Check sheet for the drawn part. Datum: minimum x, y, z corner. Units: mm. Round coordinates to 2 decimals unless told otherwise and drop trailing zeros. Write each loop counter-clockwise with the first axis right and the second up, starting at its lowest first coordinate (ties: lowest second). Pieces come first, ordered by that corner, then holes. Notation, with made-up numbers: M 47,-28.5 L 60,-28.5 A27 cw 60,10.5 Z; hole C 81,75.25 d9. An arc over 180 degrees is marked long. One line per item, written item: value. Start each with the question number.
1. Section check A-A (y = 49). Record the boundary of the cut face in (x, z).
2. Scan lines: probe 1 along Y at (x, z) = (34, 0.75) (1 decimal); probe 2 along X at (y, z) = (39.5, 1.4); probe 3 along Y at (x, z) = (31.5, 0.1) (1 decimal). Record each from-to range of solid material in increasing order. Write a range as [from, to].
3. Section check C-C (z = 1.95). Record the boundary of the cut face in (x, y) (1 decimal).
4. Section check B-B (x = 39). Record the boundary of the cut face in (y, z) (1 decimal), and give its area (3 significant figures).
5. Section check D-D (x = 19). Record the boundary of the cut face in (y, z) (1 decimal).
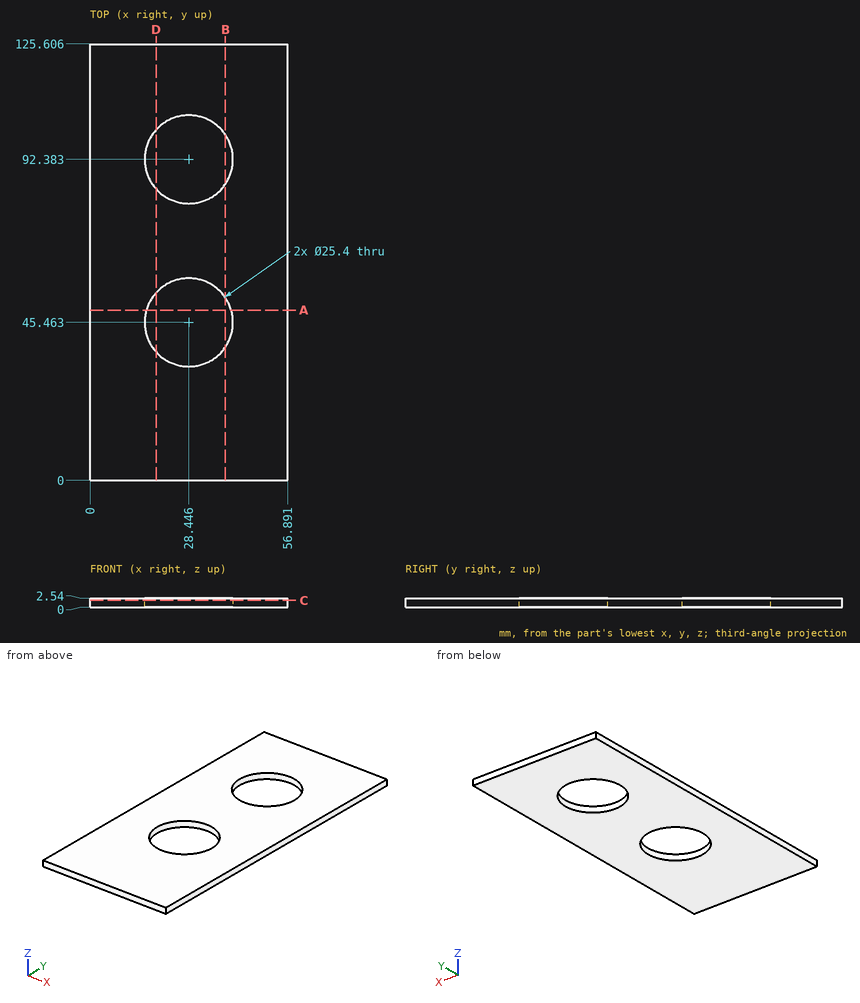
Result sheet:
1. outline: M 0,0 L 16.25,0 L 16.25,2.54 L 0,2.54 Z; M 40.64,0 L 56.89,0 L 56.89,2.54 L 40.64,2.54 Z
2. probe 1: y = [0, 34], [56.9, 81], [103.8, 125.6]
2. probe 2: x = [0, 17.23], [39.66, 56.89]
2. probe 3: y = [0, 33.1], [57.8, 80.1], [104.7, 125.6]
3. outline: M 0,0 L 56.9,0 L 56.9,125.6 L 0,125.6 Z; hole C 28.4,45.5 d25.4; hole C 28.4,92.4 d25.4
4. outline: M 0,0 L 38.4,0 L 38.4,2.5 L 0,2.5 Z; M 52.5,0 L 85.3,0 L 85.3,2.5 L 52.5,2.5 Z; M 99.4,0 L 125.6,0 L 125.6,2.5 L 99.4,2.5 Z
4. area: 247 mm2
5. outline: M 0,0 L 37,0 L 37,2.5 L 0,2.5 Z; M 54,0 L 83.9,0 L 83.9,2.5 L 54,2.5 Z; M 100.9,0 L 125.6,0 L 125.6,2.5 L 100.9,2.5 Z
